Verification items for the finished model (mm, model axes). A direction names the side the tool comes from. Coordinates: 2 decimals unless noted, no trailing zeros. Write each loop counter-clockwise with the first axis right and the second up, starting at its lowest first coordinate (ties: lowest second). Pieces come first, ordered by that corner, then holes. Notation, with made-up numbers: M -36,26.5 L -14,26.5 A12 cw -14,39.5 Z; hole C 70.5,-10.5 d4. An arc over 180 degrees is marked long. One line per item, written item: value.
Autodesk Inventor part; units mm, degrees
ref_plane "YZ Plane" through (0, 0, 0) normal (1, 0, 0) x (0, 1, 0)
ref_plane "XZ Plane" through (0, 0, 0) normal (0, 1, 0) x (-1, 0, 0)
ref_plane "XY Plane" through (0, 0, 0) normal (0, 0, 1) x (1, 0, 0)
sketch "Sketch1" plane through (0, 0, 0) normal (0, 0, 1) x (1, 0, 0)
  line L0 (-1.5978, -2.2765) -> (34.3311, -2.2765)
  line L1 (91.4022, -9.2765) -> (91.4022, -10.2765)
  line L2 (84.4022, -17.2765) -> (-1.5978, -17.2765)
  line L3 (-8.5978, -10.2765) -> (-8.5978, -9.2765)
  arc A0 (-1.5978, -2.2765) -> (-8.5978, -9.2765) centre (-1.5978, -9.2765) ccw
  arc A1 (-8.5978, -10.2765) -> (-1.5978, -17.2765) centre (-1.5978, -10.2765) ccw
  arc A2 (84.4022, -17.2765) -> (91.4022, -10.2765) centre (84.4022, -10.2765) ccw
  arc A3 (91.4022, -9.2765) -> (84.4022, -2.2765) centre (84.4022, -9.2765) ccw
  circle A4 centre (1.4022, -9.7765) radius 2.5
  circle A5 centre (81.4022, -9.7765) radius 2.5
  circle A6 centre (41.4022, -4.7765) radius 4
  arc A7 (48.4732, -2.2765) -> (34.3311, -2.2765) centre (41.4022, -4.7765) ccw
  line L4 (34.3311, -2.2765) -> (48.4732, -2.2765)
  line L5 (48.4732, -2.2765) -> (84.4022, -2.2765)
  arc A8 (34.3311, -2.2765) -> (48.4732, -2.2765) centre (41.4022, -4.7765) ccw
  point P0 (0, 0)
  point P1 (91.4022, -17.2765)
  point P2 (91.4022, -2.2765)
  point P3 (-8.5978, -17.2765)
  point P4 (41.4022, -2.2765)
  dimension "d0" = 100
  dimension "d1" = 15
  dimension "d2" = 7
  dimension "d3" = 5
  dimension "d4" = 5
  dimension "d7" = 8
  dimension "d8" = 7.5
  dimension "d9" = 7.5
  dimension "d10" = 80
  dimension "d11" = 10
  dimension "d13" = 2.5
  dimension "d14" = 40
  dimension "d16" = 15
extrude "Extrusion1" add sketch "Sketch1" along normal blind 5 contours L0 A8 L5 A3 L1 A2 L2 A1 L3 A0 | A7 L4 A6 | L4 A6 A8
equation "\"d8\" = 0.5 * d1"
properties part number "lacznik_pary_kol_V3" material "Aluminum 6061"
Item 1: Access from +Z, -Z, +X, -X, +Y, -Y to the whole of each face (thin tool, end or side, straight path). Record for faces 1 (the face through (-6.493, -15.28, 2.465)), 2 (the face through (66, -2.276, 2)), 3 (the face through (16, -2.276, 2)).
The answers:
face 1: +Z, -Z, -X, -Y
face 2: +Z, -Z, +X, +Y
face 3: +Z, -Z, -X, +Y
Item 2: Go/stop test with flat-tipped pins: P1, Ø2, axis at y = -14, z = 2.5, coming from the +X side; P2, Ø4.5, axis at x = 81.4, y = -9.78, coming from the -Z side; P3, Ø3, axis at x = 64, z = 0.5, coming from the +Y side. Record where each tip stops, or that it passes through.
The answers:
P1: stops at x = 90.85
P2: passes through
P3: stops at y = -2.28
Item 3: Cross-section at C-C, the plane x = 44. Enter the section's corners in (y, z), and give its area (3 significant figures).
The answers:
outline: M -17.28,0 L -7.82,0 L -7.82,5 L -17.28,5 Z; M -1.73,0 L 2.26,0 L 2.26,5 L -1.73,5 Z
area: 67.3 mm²
Item 4: Scan lines: line 1 (Y direction, x = 41, z = 3.6); line 2 (X direction, y = -10.25, z = 1.5); line 3 (Y direction, x = 81.5, z = 3.9). Record each from-to range of solid material in increasing order.
The answers:
line 1: y = -17.28 to -8.76, -0.8 to 2.71
line 2: x = -8.6 to -1.05, 3.86 to 78.95, 83.86 to 91.4
line 3: y = -17.28 to -12.27, -7.28 to -2.28
Item 5: Cross-section at D-D, the plane y = 1.5. Enter the section's corners in (x, z), and give its area (3 significant figures).
The answers:
outline: M 37.3,0 L 45.51,0 L 45.51,5 L 37.3,5 Z
area: 41.1 mm²
Item 6: Cross-section at A-A, the plane x = 80. Enter the section's corners in (y, z), and give its area (3 significant figures).
The answers:
outline: M -17.28,0 L -11.85,0 L -11.85,5 L -17.28,5 Z; M -7.71,0 L -2.28,0 L -2.28,5 L -7.71,5 Z
area: 54.3 mm²
Item 7: Draft check along X on faces 4 (the face through (41, -9, 5)), 5 (the face through (1.077, -12.255, 2.465)), 6 (the face through (89.41, -15.17, 2.46)), 7 (the face through (83.787, -10.527, 2.465)). Enter one of: released by +X, released by -X, zero draft, split by the parting line, or undercut.
The answers:
face 4: zero draft
face 5: undercut
face 6: released by +X
face 7: undercut
Item 8: Cross-section at B-B, the plane z = 1.9. Enter the section's corners in (x, y).
The answers:
outline: M -8.6,-10.28 A7 ccw -1.6,-17.28 L 84.4,-17.28 A7 ccw 91.4,-10.28 L 91.4,-9.28 A7 ccw 84.4,-2.28 L 48.47,-2.28 A7.5 ccw 34.33,-2.28 L -1.6,-2.28 A7 ccw -8.6,-9.28 Z; hole C 1.4,-9.78 d5; hole C 41.4,-4.78 d8; hole C 81.4,-9.78 d5
